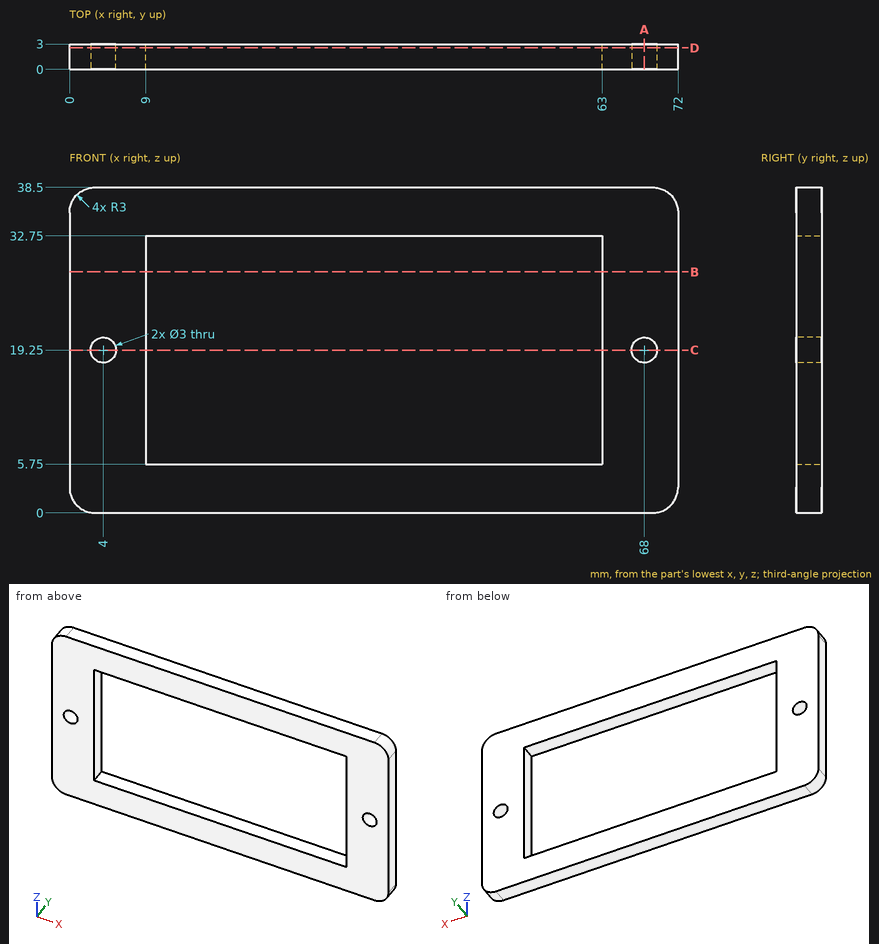
Study the drawing (mm; zero at the part's minimum x, y, z) and answer. Coordinates: 2 decimals unless noted, no trailing zeros. Write each loop counter-clockwise with the first axis right and the second up, starting at its lowest first coordinate (ties: lowest second). Pieces come first, ordered by that corner, then holes.
Q1. A cutting plane is placed at B-B, the plane z = 28.5. Give the vertices of the cut face in (x, y), then the cut area to 3 significant figures.
Q2. A cutting plane is placed at A-A, the plane x = 68. Give the vertices of the cut face in (y, z).
Q3. A cutting plane is placed at D-D, the plane y = 2.55. Give the vertices of the cut face in (x, z), then the cut area to 3 significant figures.
Q4. Find the intervals of material crossed by line 1 (X direction, y = 1.2, z = 19.25); line 2 (X direction, y = 1.9, z = 23.5); line 3 (Z direction, x = 4, y = 1.9), in increasing order.
Q5. A cutting plane is placed at C-C, the plane z = 19.25. Give the vertices of the cut face in (x, y).
Findings below:
1. outline: (0, 0) - (9, 0) - (9, 3) - (0, 3) - close; (63, 0) - (72, 0) - (72, 3) - (63, 3) - close
1. area: 54.0 mm2
2. outline: (0, 0) - (3, 0) - (3, 17.75) - (0, 17.75) - close; (0, 20.75) - (3, 20.75) - (3, 38.5) - (0, 38.5) - close
3. outline: (0, 3) arc R3 ccw to (3, 0) - (69, 0) arc R3 ccw to (72, 3) - (72, 35.5) arc R3 ccw to (69, 38.5) - (3, 38.5) arc R3 ccw to (0, 35.5) - close; hole circle Ø3 at (4, 19.25); hole (9, 5.75) - (63, 5.75) - (63, 32.75) - (9, 32.75) - close; hole circle Ø3 at (68, 19.25)
3. area: 1,290 mm2
4. line 1: x = 0 to 2.5, 5.5 to 9, 63 to 66.5, 69.5 to 72
4. line 2: x = 0 to 9, 63 to 72
4. line 3: z = 0 to 17.75, 20.75 to 38.5
5. outline: (0, 0) - (2.5, 0) - (2.5, 3) - (0, 3) - close; (5.5, 0) - (9, 0) - (9, 3) - (5.5, 3) - close; (63, 0) - (66.5, 0) - (66.5, 3) - (63, 3) - close; (69.5, 0) - (72, 0) - (72, 3) - (69.5, 3) - close
